Read the model definition and answer for the solid it produces. Units are mm, in the model's axes. A direction names the side the tool comes from. Coordinates: 2 decimals unless noted, no trailing zeros. Loops run counter-clockwise (first coordinate to the right, second up) from the corner with the lowest first, then second, coordinate; pieces in that order, holes last.
from build123d import *

# Parameters (mm, degrees)
SKETCH1_R               = 3.1
BOSS_EXTRUDE1_DEPTH     = 460
SKETCH5_R               = 4.5
CUT_EXTRUDE2_DEPTH      = 5.507107651
CUT_EXTRUDE2_DEPTH_BACK = 12


with BuildPart() as part:
    # Sketch1 → Boss-Extrude1 (new body)
    with BuildSketch(Plane.XY):
        with BuildLine():
            Line((-10, 3.1), (-8.2, 3.1))
            Line((-8.2, 3.1), (-8.2, 5.1))
            Line((-8.2, 5.1), (-6.4, 5.1))
            Line((-6.4, 5.1), (-5.492892349, 4.192892349))
            Line((-5.492892349, 4.192892349), (-5.492892349, -4.192892349))
            Line((-5.492892349, -4.192892349), (-6.4, -5.1))
            Line((-6.4, -5.1), (-8.2, -5.1))
            Line((-8.2, -5.1), (-8.2, -3.1))
            Line((-8.2, -3.1), (-10, -3.1))
            Line((-10, -3.1), (-10, -8.5))
            ThreePointArc((-10, -8.5), (-9.560660172, -9.560660172), (-8.5, -10))
            Line((-8.5, -10), (-3.1, -10))
            Line((-3.1, -10), (-3.1, -8.2))
            Line((-3.1, -8.2), (-5.1, -8.2))
            Line((-5.1, -8.2), (-5.1, -6.4))
            Line((-5.1, -6.4), (-4.192892349, -5.492892349))
            Line((-4.192892349, -5.492892349), (4.192892349, -5.492892349))
            Line((4.192892349, -5.492892349), (5.1, -6.4))
            Line((5.1, -6.4), (5.1, -8.2))
            Line((5.1, -8.2), (3.1, -8.2))
            Line((3.1, -8.2), (3.1, -10))
            Line((3.1, -10), (8.5, -10))
            ThreePointArc((8.5, -10), (9.560660172, -9.560660172), (10, -8.5))
            Line((10, -8.5), (10, -3.1))
            Line((10, -3.1), (8.2, -3.1))
            Line((8.2, -3.1), (8.2, -5.1))
            Line((8.2, -5.1), (6.4, -5.1))
            Line((6.4, -5.1), (5.492892349, -4.192892349))
            Line((5.492892349, -4.192892349), (5.492892349, 4.192892349))
            Line((5.492892349, 4.192892349), (6.4, 5.1))
            Line((6.4, 5.1), (8.2, 5.1))
            Line((8.2, 5.1), (8.2, 3.1))
            Line((8.2, 3.1), (10, 3.1))
            Line((10, 3.1), (10, 8.5))
            ThreePointArc((10, 8.5), (9.560660172, 9.560660172), (8.5, 10))
            Line((8.5, 10), (3.1, 10))
            Line((3.1, 10), (3.1, 8.2))
            Line((3.1, 8.2), (5.1, 8.2))
            Line((5.1, 8.2), (5.1, 6.4))
            Line((5.1, 6.4), (4.192892349, 5.492892349))
            Line((4.192892349, 5.492892349), (-4.192892349, 5.492892349))
            Line((-4.192892349, 5.492892349), (-5.1, 6.4))
            Line((-5.1, 6.4), (-5.1, 8.2))
            Line((-5.1, 8.2), (-3.1, 8.2))
            Line((-3.1, 8.2), (-3.1, 10))
            Line((-3.1, 10), (-8.5, 10))
            ThreePointArc((-8.5, 10), (-9.560660172, 9.560660172), (-10, 8.5))
            Line((-10, 8.5), (-10, 3.1))
        make_face()
        Circle(SKETCH1_R, mode=Mode.SUBTRACT)
    extrude(amount=BOSS_EXTRUDE1_DEPTH)

    # Sketch5 → Cut-Extrude2 (cut, two sides)
    with BuildSketch(Plane(origin=(-5.492892349, 0, 0), x_dir=(0, 0, -1), z_dir=(-1, 0, 0))) as cut_extrude2_sk:
        with Locations((-230, 0)):
            Circle(SKETCH5_R)
    extrude(amount=CUT_EXTRUDE2_DEPTH, mode=Mode.SUBTRACT)
    extrude(cut_extrude2_sk.sketch, amount=-CUT_EXTRUDE2_DEPTH_BACK, mode=Mode.SUBTRACT)


solid = part.part
Q1. Determine the mould class of faces 1 (the face through (-5.493, 0, 344)), 2 (the face through (0, 5.493, 227)), 3 (the face through (-2.4, 2.4, 0)) for opening direction Y: +Y half, -Y half, draft (parallel to the pull), parting line (faces both ways), or undercut.
Findings below:
face 1: undercut
face 2: undercut
face 3: draft
Q2. A cutting plane is placed at B-B (x = 0). Give the vertices of the cut face in (y, z), then the cut area to 3 significant figures.
Findings below:
outline: (-5.49, 0) - (-3.1, 0) - (-3.1, 226.74) arc R4.5 cw to (-3.1, 233.26) - (-3.1, 460) - (-5.49, 460) - close; (3.1, 0) - (5.49, 0) - (5.49, 460) - (3.1, 460) - (3.1, 233.26) arc R4.5 cw to (3.1, 226.74) - close
area: 2,190 mm2
Q3. A cutting plane is placed at A-A (y = 0). Give the vertices of the cut face in (x, z), then the cut area to 3 significant figures.
Findings below:
outline: (-5.49, 0) - (-3.1, 0) - (-3.1, 225.5) - (-5.49, 225.5) - close; (-5.49, 234.5) - (-3.1, 234.5) - (-3.1, 460) - (-5.49, 460) - close; (3.1, 0) - (5.49, 0) - (5.49, 225.5) - (3.1, 225.5) - close; (3.1, 234.5) - (5.49, 234.5) - (5.49, 460) - (3.1, 460) - close
area: 2,160 mm2
Q4. Straight lines are drawn through the part: probe 1 along X at (y, z) = (-3.25, 187); probe 2 along X at (y, z) = (-7, 78); probe 3 along Y at (x, z) = (0, 411). For each, find the intervals that lie inside material, in ascending order.
Findings below:
probe 1: x = -10 to -8.2, -5.49 to 5.49, 8.2 to 10
probe 2: x = -10 to -5.1, 5.1 to 10
probe 3: y = -5.49 to -3.1, 3.1 to 5.49
Q5. Flat-ended cylindrical pins translate along their axes: pin 1 Ø6 at (x, z) = (1.5, 398) entering from -Y; pin 2 Ø2.5 at (x, z) = (-1.5, 285.5) entering from +Y; pin 3 Ø1.5 at (y, z) = (0.5, 186) entering from -X; pin 4 Ø4 at (y, z) = (1, 77) entering from +X. Find the tip coordinate at first contact, or state that the pin passes through.
Findings below:
pin 1: stops at y = -10
pin 2: stops at y = 5.49
pin 3: stops at x = -5.49
pin 4: stops at x = 5.49
Q6. Which of the six approach directions +Z, -Z, +X, -X, +Y, -Y give full straight-line access (tool end or side, diameter ignored) to faces 4 (the face through (0, -5.493, 227)), 5 (the face through (-2.4, 2.4, 460))?
Findings below:
face 4: +Z, -Z
face 5: +Z, +X, -X, +Y, -Y
